Could you check a few things on this model? Use its own coordinates, in mm. A direction names the side the tool comes from. Give positions to 0.01 mm unless a question says otherwise; leave off trailing zeros. Loops run counter-clockwise (first coordinate to the right, second up) from the corner with the lowest first, then second, coordinate; pieces in that order, holes last. Notation, with made-up numbers: M -3.75,-37.5 L 29.25,-37.5 A27 ccw 29.25,-5.5 Z; hole C -16.75,38 d2. An arc over 180 degrees is marked long. Use CSV: the item, a comma, the result in double quotes.
```python
from build123d import *

# Parameters (mm, degrees)
F1_DEPTH = 17.4625
F3_D     = 9.8425
F4_R     = 5.08
F6_D     = 9.525
F7_R     = 5.08


with BuildPart() as f1:
    # F0 (on Top) → F1 (new body)
    with BuildSketch(Plane.XY):
        Polygon((-31.75, -63.5), (31.75, -63.5), (31.75, -44.45), (6.35, -44.45), (6.35, 44.45), (31.75, 44.45), (31.75, 63.5), (-31.75, 63.5), align=None)
    extrude(amount=F1_DEPTH)

    # F3 (through all)
    with Locations(Plane(origin=(0, 63.5, 0), x_dir=(-1, 0, 0), z_dir=(0, 1, 0))):
        with Locations((-22.225, 8.73125)):
            Hole(F3_D / 2)

    # F4
    f4_edges = [f1.edges().sort_by_distance(p)[0] for p in [
        (6.35, -44.45, 8.73125),
        (6.35, 44.45, 8.73125),
    ]]
    fillet(f4_edges, radius=F4_R)

    # F6 (through all)
    with Locations(Plane(origin=(0, 0, 0), x_dir=(1, 0, 0), z_dir=(0, 0, -1))):
        with Locations((-12.7, 38.1), (-12.7, -38.1)):
            Hole(F6_D / 2)

    # F7
    f7_edges = [f1.edges().sort_by_distance(p)[0] for p in [
        (31.75, -53.975, 17.4625),
        (31.75, -53.975, 0),
        (31.75, 53.975, 17.4625),
        (31.75, 53.975, 0),
    ]]
    fillet(f7_edges, radius=F7_R)


solid = f1.part
```
1. I want a section at D-D, the plane x = 19.5. List the corners of the cut face in (y, z) for me, then the cut area to 3 significant figures.
Outcome:
outline,"M -63.5,0 L -44.45,0 L -44.45,4.63 L -63.5,4.63 Z; M -63.5,12.83 L -44.45,12.83 L -44.45,17.46 L -63.5,17.46 Z; M 44.45,0 L 63.5,0 L 63.5,4.63 L 44.45,4.63 Z; M 44.45,12.83 L 63.5,12.83 L 63.5,17.46 L 44.45,17.46 Z"
area,"353 mm2"
2. If we mould it in two halves opening along Y, with no side actions, what happens to faces 1 (the face through (0, 63.5, 9)), 2 (the face through (30.301, 54.108, 15.935)), 3 (the face through (-8.92, -35.2, 8.85))? For each: +Y half, -Y half, draft (parallel to the pull), parting line (faces both ways), or undercut.
Outcome:
face 1,"+Y half"
face 2,"draft"
face 3,"undercut"
3. I want a section at B-B, the plane y = -38.1. List the corners of the cut face in (x, z) for me.
Outcome:
outline,"M -31.75,0 L -17.46,0 L -17.46,17.46 L -31.75,17.46 Z; M -7.94,0 L 6.35,0 L 6.35,17.46 L -7.94,17.46 Z"
4. I want a section at A-A, the plane x = -12.7. List the corners of the cut face in (y, z) for me.
Outcome:
outline,"M -63.5,0 L -42.86,0 L -42.86,17.46 L -63.5,17.46 Z; M -33.34,0 L 33.34,0 L 33.34,17.46 L -33.34,17.46 Z; M 42.86,0 L 63.5,0 L 63.5,17.46 L 42.86,17.46 Z"
5. I'm going to push flat-ended pins straight in: pin 1 Ø3 at (y, z) = (44.5, 14.5) entering from +X; pin 2 Ø8 at (x, z) = (22.22, 8.73) entering from +Y. Where does each tip first touch, or does it pass through?
Outcome:
pin 1,"x = 31.71"
pin 2,"through"
6. Which directions (+Z, -Z, +X, -X, +Y, -Y) give clear straight access to the entire face, cutting with the end or side of a thin tool? Please do faces 4 (the face through (6.35, -1, 9)), 5 (the face through (30.301, -53.842, 15.935)).
Outcome:
face 4,"+Z, -Z, +X"
face 5,"+Z, +X, +Y, -Y"
7. I want a section at C-C, the plane z = 15. Give the number of separate pieces and of enclosed holes in the cut face, then the cut area to 3 significant figures.
Outcome:
separate pieces,"1"
enclosed holes,"2"
area,"5,650 mm2"
8. Please list where these lines run through material, in increasing order: line 1 (Y direction, x = -12.7, z = 12); line 2 (X direction, y = -38.5, z = 4); line 3 (Y direction, x = -11.5, z = 5.5).
Outcome:
line 1,"-63.5 to -42.86, -33.34 to 33.34, 42.86 to 63.5"
line 2,"-31.75 to -17.45, -7.95 to 6.35"
line 3,"-63.5 to -42.71, -33.49 to 33.49, 42.71 to 63.5"
